from build123d import *

# Parameters (mm, degrees)
F0_R          = 12.7
F1_DEPTH      = 38.1
F1_DEPTH_BACK = 38.1
F2_R          = 1.651
F3_DEPTH      = 12.7


with BuildPart() as f1:
    # F0 (on Right) → F1 (new body, two sides)
    with BuildSketch(Plane.YZ) as f1_sk:
        with BuildLine():
            Line((19.05, 0), (19.05, 25.4))
            ThreePointArc((19.05, 25.4), (0, 44.45), (-19.05, 25.4))
            Line((-19.05, 25.4), (-19.05, 0))
            Line((-19.05, 0), (19.05, 0))
        make_face()
        with Locations((0, 25.4)):
            Circle(F0_R, mode=Mode.SUBTRACT)
    extrude(amount=F1_DEPTH)
    extrude(f1_sk.sketch, amount=-F1_DEPTH_BACK)

    # F2 (on face) → F3 (cut)
    with BuildSketch(Plane(origin=(0, 0, 0), x_dir=(1, 0, 0), z_dir=(0, 0, -1))):
        with Locations((-31.75, 12.7)):
            Circle(F2_R)
        with Locations((-31.75, -12.7)):
            Circle(F2_R)
        with Locations((31.75, 12.7)):
            Circle(F2_R)
        with Locations((31.75, -12.7)):
            Circle(F2_R)
    extrude(amount=-F3_DEPTH, mode=Mode.SUBTRACT)


solid = f1.part
Verification items for the finished model (mm, model axes). A direction names the side the tool comes from. Coordinates: 2 decimals unless noted, no trailing zeros. Write each loop counter-clockwise with the first axis right and the second up, starting at its lowest first coordinate (ties: lowest second). Pieces come first, ordered by that corner, then holes. Notation, with made-up numbers: M 52,81 L 91,81 A28 cw 91,102 Z; hole C -31.5,88 d1. An arc over 180 degrees is marked long. Use a Markdown table: item, result.
Q1. Go/stop test with flat-tipped pins: P1, Ø2, axis at x = 31.75, y = 12.7, coming from the +Z side; P2, Ø2.5, axis at x = 31.75, y = -12.7, coming from the +Z side (3 decimals); P3, Ø1, axis at x = 31, y = -12, coming from the -Z side. Record where each tip stops, or that it passes through.
Reply:
| item | result |
|---|---|
| P1 | stops at z = 40.43 |
| P2 | stops at z = 40.625 |
| P3 | stops at z = 12.7 |
Q2. Sectioned sample at B-B, the plane x = 31.75. Record the boundary of the cut face in (y, z), plus the area to 3 significant figures.
Reply:
| item | result |
|---|---|
| outline | M -19.05,0 L -14.35,0 L -14.35,12.7 L -11.05,12.7 L -11.05,0 L 11.05,0 L 11.05,12.7 L 14.35,12.7 L 14.35,0 L 19.05,0 L 19.05,25.4 A19.05 ccw -19.05,25.4 Z; hole C 0,25.4 d25.4 |
| area | 947 mm² |
Q3. Sectioned sample at D-D, the plane x = -2. Record the boundary of the cut face in (y, z).
Reply:
| item | result |
|---|---|
| outline | M -19.05,0 L 19.05,0 L 19.05,25.4 A19.05 ccw -19.05,25.4 Z; hole C 0,25.4 d25.4 |
Q4. Sectioned sample at C-C, the plane z = 17. Record the boundary of the cut face in (x, y), plus the area to 3 significant figures.
Reply:
| item | result |
|---|---|
| outline | M -38.1,-19.05 L 38.1,-19.05 L 38.1,-9.53 L -38.1,-9.53 Z; M -38.1,9.53 L 38.1,9.53 L 38.1,19.05 L -38.1,19.05 Z |
| area | 1,450 mm² |
Q5. Draft check along X on faces 1 (the face through (0.533, 0.419, 44.445)), 2 (the face through (-31.965, -14.337, 6.261)), 3 (the face through (-38.1, -5, 13)). Enter one of: +X half, -X half, draft (parallel to the pull), parting line (faces both ways), or undercut.
Reply:
| item | result |
|---|---|
| face 1 | draft |
| face 2 | undercut |
| face 3 | -X half |
Q6. Thickness scan on line 1 (X direction, y = -12.7, z = 8.5); line 2 (Z direction, x = 14, y = 0); line 3 (Y direction, x = -31, z = 7). Record the ranges inside material, lowest first.
Reply:
| item | result |
|---|---|
| line 1 | x = -38.1 to -33.4, -30.1 to 30.1, 33.4 to 38.1 |
| line 2 | z = 0 to 12.7, 38.1 to 44.45 |
| line 3 | y = -19.05 to -14.17, -11.23 to 11.23, 14.17 to 19.05 |
Q7. Sectioned sample at A-A, the plane y = 0. Record the boundary of the cut face in (x, z).
Reply:
| item | result |
|---|---|
| outline | M -38.1,0 L 38.1,0 L 38.1,12.7 L -38.1,12.7 Z; M -38.1,38.1 L 38.1,38.1 L 38.1,44.45 L -38.1,44.45 Z |
Q8. Set-up check for faces 4 (the face through (1, 0, 0)), 5 (the face through (32, 13, 12.7)): record each of +Z, -Z, +X, -X, +Y, -Y from which the full face is reachable in a straight line by a thin tool's end or side.
Reply:
| item | result |
|---|---|
| face 4 | -Z, +X, -X, +Y, -Y |
| face 5 | -Z |
